Job drawing, mm, ordinate dimensions from the low corner. One solid piece. A direction names the side the tool comes from. Coordinates: 2 decimals unless noted, no trailing zeros. Order: outer loops, then holes, each group sorted by start corner. A loop starts at its lowest first (then second) coordinate and runs counter-clockwise, first axis right, second up. Notation, with made-up numbers: (62.5, 41) -> (76.5, 41) arc R11 ccw to (76.5, 56) -> close; hole circle Ø1 at (63, 14.25). An arc over 180 degrees is marked (long way). Use CSV: the item, a comma, the result in double quotes. Start each with the question number.
(1) Cut at D-D on y = 9.25. Write the cut outline in (x, z), plus the area to 3 significant figures.
(2) Pin check, flat tips, straight feed: pin 1 Ø4 at (x, z) = (45.5, 19.5) entering from -Y; pin 2 Ø1 at (y, z) = (4, 7.5) entering from -X; pin 3 Ø2.5 at (x, y) = (4.35, 5) entering from +Z; pin 4 Ø1 at (y, z) = (6, 6.5) entering from +X. Stop position of each tip, or through.
(3) Cut at B-B on x = 38. Write the cut outline in (y, z), plus the area to 3 significant figures.
(4) Probe L1, parallel to Y at x = 4.35, z = 21.25; L2, parallel to X at y = 9, z = 1.25; L3, parallel to Z at x = 39.5, y = 2.25. List the from-to ranges inside material, lowest first.
(5) Pull direction X, two halves, no side cores. Call the marked faces 4, 5 and 6: pulls with the +X half, pulls with the -X half, needs draft (parallel to the pull), parting line crosses it, or undercut.
(6) Tool access for the marked faces 1, 2 and 3: list every direction of +Z, -Z, +X, -X, +Y, -Y with a clear straight run to the whole face (end or side of a thin tool).
(7) Cut at A-A on z = 4. Write the cut outline in (x, y), plus the area to 3 significant figures.
(8) Cut at C-C on x = 46.65. Write the cut outline in (y, z), plus the area to 3 significant figures.
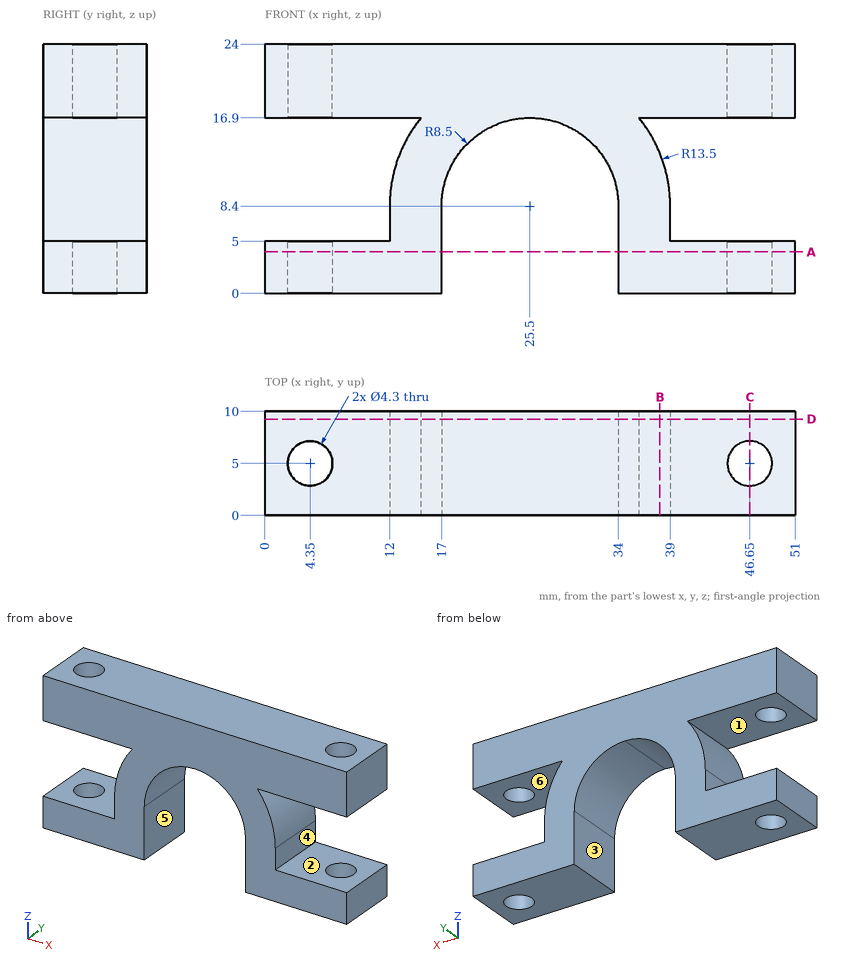
Outcome:
1,outline,"(0, 0) -> (17, 0) -> (17, 8.4) arc R8.5 cw to (34, 8.4) -> (34, 0) -> (51, 0) -> (51, 5) -> (39, 5) -> (39, 8.4) arc R13.5 ccw to (35.99, 16.9) -> (51, 16.9) -> (51, 24) -> (0, 24) -> (0, 16.9) -> (15.01, 16.9) arc R13.5 ccw to (12, 8.4) -> (12, 5) -> (0, 5) -> close"
1,area,"666 mm2"
2,pin 1,"y = 0"
2,pin 2,"x = 12"
2,pin 3,"through"
2,pin 4,"x = 39"
3,outline,"(0, 0) -> (10, 0) -> (10, 13.5) -> (0, 13.5) -> close; (0, 16.9) -> (10, 16.9) -> (10, 24) -> (0, 24) -> close"
3,area,"206 mm2"
4,L1,"0 to 2.85, 7.15 to 10"
4,L2,"0 to 17, 34 to 51"
4,L3,"0 to 5, 16.9 to 24"
5,face 4,"pulls with the +X half"
5,face 5,"undercut"
5,face 6,"needs draft"
6,face 1,"-X, +Y, -Y"
6,face 2,"+X, +Y, -Y"
6,face 3,"-Z, +Y, -Y"
7,outline,"(0, 0) -> (17, 0) -> (17, 10) -> (0, 10) -> close; (34, 0) -> (51, 0) -> (51, 10) -> (34, 10) -> close; hole circle Ø4.3 at (4.35, 5); hole circle Ø4.3 at (46.65, 5)"
7,area,"311 mm2"
8,outline,"(0, 0) -> (2.85, 0) -> (2.85, 5) -> (0, 5) -> close; (0, 16.9) -> (2.85, 16.9) -> (2.85, 24) -> (0, 24) -> close; (7.15, 0) -> (10, 0) -> (10, 5) -> (7.15, 5) -> close; (7.15, 16.9) -> (10, 16.9) -> (10, 24) -> (7.15, 24) -> close"
8,area,"69.0 mm2"
